Autodesk Inventor part; units mm, degrees
ref_plane "YZ Plane" through (0, 0, 0) normal (1, 0, 0) x (0, 1, 0)
ref_plane "XZ Plane" through (0, 0, 0) normal (0, 1, 0) x (-1, 0, 0)
ref_plane "XY Plane" through (0, 0, 0) normal (0, 0, 1) x (1, 0, 0)
sketch "Sketch1" plane through (0, 0, 0) normal (1, 0, 0) x (0, 1, 0)
  line L0 (0, 0) -> (30, 0)
  line L1 (30, 0) -> (30, -20)
  line L2 (30, -20) -> (0, -20)
  line L3 (0, -20) -> (0, 0)
  dimension "d0" = 30
  dimension "d1" = 20
extrude "Extrusion1" add sketch "Sketch1" along normal blind 30
sketch "Sketch2" plane through (0, 30, 0) normal (0, 1, 0) x (1, 0, 0)
  line L0 (0, 0) -> (30, 0)
  line L1 (0, 20) -> (30, 20)
  line L2 (5, 0) -> (25, 0)
  line L3 (25, 0) -> (25, 20)
  line L4 (25, 20) -> (5, 20)
  line L5 (5, 20) -> (5, 0)
  line L6 (30, 20) -> (30, 0)
  dimension "d4" = 5
  dimension "d5" = 5
extrude "Extrusion2" cut sketch "Sketch2" against normal blind 25 contours L5 L1 L3 L0
fillet "Fillet1" radius 2.5 2 edges at (5, 5, -10) (25, 5, -10)
hole "Hole1" at (0, 20, -10) direction (1, 0, 0) diameter 12 end through all
fillet "Fillet3" radius 10 4 edges at (27.5, 30, -20) (2.5, 30, -20) (2.5, 30, 0) (27.5, 30, 0)
sketch "Sketch4" plane through (0, 5, 0) normal (0, 1, 0) x (1, 0, 0)
  line L0 (0, 4) -> (0, 16)
  line L1 (0, 10) -> (30, 10)
  line L2 (30, 20) -> (30, 0)
  point P0 (0, 0)
  point P1 (15, 10)
hole "Hole2" at (15, 5, -10) direction (0, -1, 0) diameter 9 end through all
properties part number "Damper_Mount_03"
Check sheet for the modelled part. Datum: model origin and axes. Units: mm. A direction names the side the tool comes from. Coordinates: 2 decimals unless noted, no trailing zeros. Write each loop counter-clockwise with the first axis right and the second up, starting at its lowest first coordinate (ties: lowest second). Pieces come first, ordered by that corner, then holes. Notation, with made-up numbers: M -30.75,-3 L -15.75,-3 A29 ccw -15.75,33 Z; hole C 9,8.25 d1. An arc over 180 degrees is marked long. Write item = value, one per line. Start each with the question number.
1. Sectioned sample at B-B (z = -12.75). Record the cut outline in (x, y).
2. Tool access check on faces 4 (the cylindrical face through (27.54, 26.99, -17.15)), 5 (the flat face through (15, 5, -15)). Record the directions out of +Z, -Z, +X, -X, +Y, -Y that give a thin tool (end or side, any length) a straight path to the whole face; none if there is none.
3. Go/stop test with flat-tipped pins: pin 1 (5.5 mm diameter, centred on x = 15, z = -10, fed in from +Y); pin 2 (6 mm diameter, centred on x = 18.5, z = -7, fed in from +Y); pin 3 (8 mm diameter, centred on x = 23.5, z = -5.5, fed in from +Y). Record where each tip stops, or that it passes through.
4. Mould release check, pull along X, two halves, no side actions. Record for faces 1 (the flat face through (30, 11, -10)), 2 (the flat face through (25, 14, -8)), 3 (the flat face through (15, 3, 0)): pulls with the +X half, pulls with the -X half, needs draft (parallel to the pull), parting line crosses it, or undercut.
5. Thickness scan on probe 1 along X at (y, z) = (11.75, -9); probe 2 along Z at (x, y) = (15, 2.7); probe 3 along Z at (x, y) = (3.95, 20). Record the ranges inside material, lowest first.
6. Sectioned sample at A-A (x = 15). Record the cut outline in (y, z), then the cut area to 3 significant figures.
7. Sectioned sample at D-D (y = 19.25). Record the cut outline in (x, z).
The answers:
q1.outline = M 0,0 L 11.44,0 L 11.44,5 L 7.5,5 A2.5 cw 5,7.5 L 5,14.67 L 0,14.67 Z; M 0,25.33 L 5,25.33 L 5,29.61 L 0,29.61 Z; M 18.56,0 L 30,0 L 30,14.67 L 25,14.67 L 25,7.5 A2.5 cw 22.5,5 L 18.56,5 Z; M 25,25.33 L 30,25.33 L 30,29.61 L 25,29.61 Z
q2.face_4 = -Z, +X, -X, +Y
q2.face_5 = +Z, -Z, +Y
q3.pin_1 = through
q3.pin_2 = 5
q3.pin_3 = 29.97
q4.face_1 = pulls with the +X half
q4.face_2 = undercut
q4.face_3 = needs draft
q5.probe_1 = 0 to 5, 25 to 30
q5.probe_2 = -20 to -14.5, -5.5 to 0
q5.probe_3 = -20 to -16, -4 to 0
q6.outline = M 0,-20 L 5,-20 L 5,-14.5 L 0,-14.5 Z; M 0,-5.5 L 5,-5.5 L 5,0 L 0,0 Z
q6.area = 55.0 mm²
q7.outline = M 0,-20 L 5,-20 L 5,-15.95 L 0,-15.95 Z; M 0,-4.05 L 5,-4.05 L 5,0 L 0,0 Z; M 25,-20 L 30,-20 L 30,-15.95 L 25,-15.95 Z; M 25,-4.05 L 30,-4.05 L 30,0 L 25,0 Z
